```python
from build123d import *

# Parameters (mm, degrees)
SKETCH1_R           = 29.0449
BOSS_EXTRUDE3_DEPTH = 25.4
SKETCH6_R           = 29.0449
BOSS_EXTRUDE4_DEPTH = 38.1
BOSS_EXTRUDE4_DRAFT = -35
FILLET1_R           = 25.4
SHELL2_T            = -0.762


with BuildPart() as part:
    # Sketch1 → Boss-Extrude3 (new body)
    with BuildSketch(Plane(origin=(0, 0, 0), x_dir=(1, 0, 0), z_dir=(0, 1, 0))):
        with Locations(Location((0, 0, 0), (0, 0, 270))):
            Circle(SKETCH1_R)
    extrude(amount=BOSS_EXTRUDE3_DEPTH)


with BuildPart() as boss_extrude4_tool:
    # Sketch6 → Boss-Extrude4 (with draft: the straight prism first)
    with BuildSketch(Plane(origin=(0, 25.4, 0), x_dir=(1, 0, 0), z_dir=(0, 1, 0))):
        with Locations(Location((0, 0, 0), (0, 0, 270))):
            Circle(SKETCH6_R)
    extrude(amount=BOSS_EXTRUDE4_DEPTH)
    # Boss-Extrude4: the draft: its side faces are tilted about the plane it starts from
    boss_extrude4_sides = [boss_extrude4_tool.faces().sort_by_distance(p)[0] for p in [
        (0, 44.45, -29.0449),
    ]]
    draft(boss_extrude4_sides, Plane(origin=(0, 25.4, 0), x_dir=(1, 0, 0), z_dir=(0, 1, 0)), BOSS_EXTRUDE4_DRAFT)


with BuildPart() as part_1:
    add(part.part)

    # Boss-Extrude4: add boss_extrude4_tool
    add(boss_extrude4_tool.part)

    # Fillet1
    fillet1_edges = [part_1.edges().sort_by_distance(p)[0] for p in [
        (0, 25.4, -29.0449),
    ]]
    fillet(fillet1_edges, radius=FILLET1_R)

    # Shell2
    shell2_openings = [part_1.faces().sort_by_distance(p)[0] for p in [
        (0, 0, 0),
        (0, 63.5, 0),
    ]]
    offset(amount=SHELL2_T, openings=shell2_openings, kind=Kind.INTERSECTION)


solid = part_1.part
```
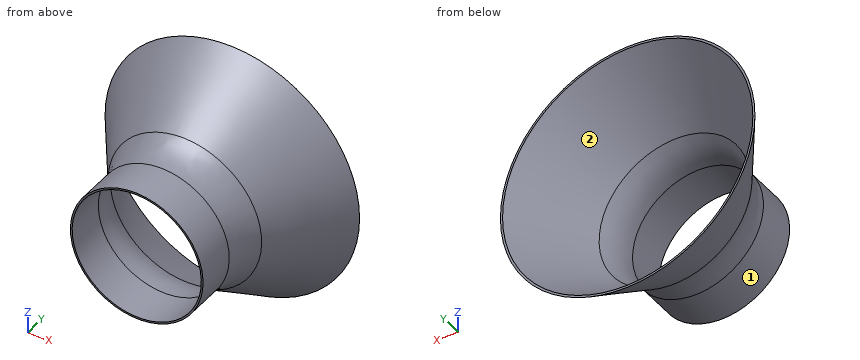
Can you work these out from the model? Positions are in its coordinate system, mm. Face numbers are marked on the shaded views. Give positions to 0.01 mm unless a question says otherwise; leave off trailing zeros. Loops run counter-clockwise (first coordinate to the right, second up) from the corner with the lowest first, then second, coordinate; pieces in that order, holes last. Notation, with made-up numbers: M 38.25,60.5 L 71.25,60.5 A3 cw 71.25,64.5 Z; hole C 4,-21.5 d6. An arc over 180 degrees is marked long. Use one line per item in the form item = value. Start each with the question number.
(1) I'm going to push flat-ended pins straight in: P1, Ø3, axis at y = 11, z = 16, coming from the +X side; P2, Ø8, axis at x = -40.5, z = 25.5, coming from the -Y side; P3, Ø6, axis at x = -15, y = 39, coming from the +Z side. Where does each tip first touch, or does it pass through?
(2) I want a section at A-A, the plane y = 38.5. Write out the boundary of the cut face in (x, z), and give its area (3 significant figures).
(3) I want a section at B-B, the plane y = 48. Write out the boundary of the cut face in (x, z), and give its area (3 significant figures).
(4) Thinking about a two-plate mould opening in X: for the marked faces 1 and 2, which applies, released by +X, released by -X, zero draft, split by the parting line, or undercut?
(5) Please list where these lines run through material, in increasing order: line 1 (Z direction, x = 0, y = 5.75); line 2 (X direction, y = 27, z = -15.5).
Worked out:
q1.P1 = 25.17
q1.P2 = 46.56
q1.P3 = 38.07
q2.outline = C 0,0 d76.44; hole C 0,0 d74.57
q2.area = 221 mm²
q3.outline = C 0,0 d89.74; hole C 0,0 d87.88
q3.area = 260 mm²
q4.face_1 = split by the parting line
q4.face_2 = undercut
q5.line_1 = -29.04 to -28.28, 28.28 to 29.04
q5.line_2 = -26.77 to -25.82, 25.82 to 26.77
